For this review, use the dimensioned drawing (mm, ordinates from the lowest corner) and the shaded views. Give positions to 0.01 mm unless a question says otherwise; leave off trailing zeros. Loops run counter-clockwise (first coordinate to the right, second up) from the corner with the lowest first, then second, coordinate; pieces in that order, holes last. Notation, with made-up numbers: (2.25, -13.5) -> (32.25, -13.5) arc R18 ccw to (32.25, -7.5) -> close; hole circle Ø5 at (-15, 22). An arc over 180 degrees is marked (long way). Write each question's results on one line, items separated by ' | '. Start each with the question number.
Q1. We need section D-D (x = 40.5). Write out the cut boundary in (y, z), plus the area to 4 significant figures.
Q2. We need section A-A (z = 3). Write out the cut boundary in (x, y), plus the area to 3 significant figures.
Q3. We need section B-B (x = 3). Write out the cut boundary in (y, z), plus the area to 3 significant figures.
Q4. Wall thickness on L1, parallel to Z at x = 41, y = 2.8; L2, parallel to X at y = 0.6, z = 3; L3, parallel to Z at x = 33.5, y = 1.15: over which ranges is each line inside the solid? List them lowest first. Write a range as [from, to].
Q5. Mouldability with a two-part tool opening along Y and no side actions: class the marked faces 1 and 2 as released by +Y, released by -Y, zero draft, split by the parting line, or undercut.
Q6. We need section C-C (z = 26.5). Write out the cut boundary in (x, y), plus the area to 3 significant figures.
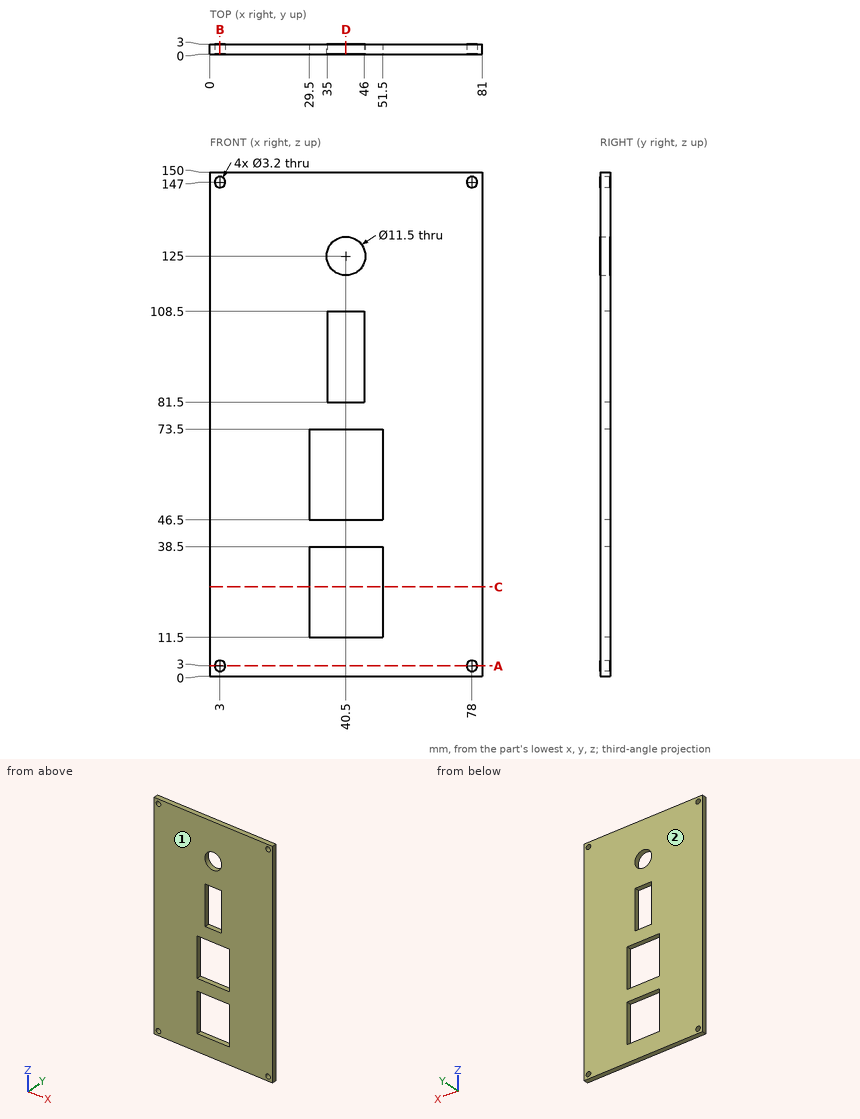
Output:
1) outline: (0, 0) -> (3, 0) -> (3, 11.5) -> (0, 11.5) -> close; (0, 38.5) -> (3, 38.5) -> (3, 46.5) -> (0, 46.5) -> close; (0, 73.5) -> (3, 73.5) -> (3, 81.5) -> (0, 81.5) -> close; (0, 108.5) -> (3, 108.5) -> (3, 119.25) -> (0, 119.25) -> close; (0, 130.75) -> (3, 130.75) -> (3, 150) -> (0, 150) -> close | area: 172.5 mm2
2) outline: (0, 0) -> (1.4, 0) -> (1.4, 3) -> (0, 3) -> close; (4.6, 0) -> (76.4, 0) -> (76.4, 3) -> (4.6, 3) -> close; (79.6, 0) -> (81, 0) -> (81, 3) -> (79.6, 3) -> close | area: 224 mm2
3) outline: (0, 0) -> (3, 0) -> (3, 1.4) -> (0, 1.4) -> close; (0, 4.6) -> (3, 4.6) -> (3, 145.4) -> (0, 145.4) -> close; (0, 148.6) -> (3, 148.6) -> (3, 150) -> (0, 150) -> close | area: 431 mm2
4) L1: [0, 11.5], [38.5, 46.5], [73.5, 81.5], [108.5, 119.27], [130.73, 150] | L2: [0, 1.4], [4.6, 76.4], [79.6, 81] | L3: [0, 11.5], [38.5, 46.5], [73.5, 150]
5) face 1: released by -Y | face 2: released by +Y
6) outline: (0, 0) -> (29.5, 0) -> (29.5, 3) -> (0, 3) -> close; (51.5, 0) -> (81, 0) -> (81, 3) -> (51.5, 3) -> close | area: 177 mm2
